Could you check a few things on this model? Use its own coordinates, in mm. A direction names the side the tool comes from. Round coordinates to 2 decimals unless told otherwise and drop trailing zeros. Loops run counter-clockwise (first coordinate to the right, second up) from the corner with the lowest first, then second, coordinate; pieces in that order, holes last. Notation, with made-up numbers: (59.5, 82.25) - (72.5, 82.25) arc R12 ccw to (72.5, 87.25) - close; hole circle Ø7 at (57, -32.5). An arc over 180 degrees is marked (long way). Use one line per item in the form item = value.
```python
from build123d import *

# Parameters (mm, degrees)
SKETCH1_W                = 51
SKETCH1_H                = 53.5
BOSS_EXTRUDE1_DEPTH      = 54.25
SKETCH2_W                = 43
SKETCH2_H                = 43
CUT_EXTRUDE1_DEPTH       = 50.75
SKETCH3_W                = 43
SKETCH3_H                = 3.5
CUT_EXTRUDE2_DEPTH       = 37.5
CUT_EXTRUDE3_DEPTH       = 76
SKETCH5_R                = 9.673114497
SKETCH5_R_2              = 5.390775308
SKETCH5_R_3              = 5.456912487
CUT_EXTRUDE4_DEPTH       = 76
SKETCH6_R                = 14
SKETCH6_R_2              = 1.75
CUT_EXTRUDE5_DEPTH       = 76
SKETCH7_R                = 5
CUT_EXTRUDE6_DEPTH       = 76
CUT_EXTRUDE7_DEPTH       = 27
FILLET2_R                = 1
SKETCH12_R               = 1.75
CUT_EXTRUDE8_DEPTH       = 15
BOSS_EXTRUDE4_DEPTH      = 10
BOSS_EXTRUDE4_DEPTH_BACK = 61
SKETCH13_W               = 16.75
SKETCH13_H               = 3.5
SKETCH14_W               = 71
SKETCH14_H               = 1.75
BOSS_EXTRUDE5_DEPTH      = 15
SKETCH15_R               = 1.75
CUT_EXTRUDE9_DEPTH       = 10
SKETCH16_R               = 1.75
CUT_EXTRUDE10_DEPTH      = 10
CUT_EXTRUDE11_REACH      = 95.245
FILLET3_R                = 5
FILLET4_R                = 1
CUT_EXTRUDE12_DEPTH      = 3


with BuildPart() as part:
    # Sketch1 → Boss-Extrude1 (new body)
    with BuildSketch(Plane.XY):
        with Locations((-26.432354029, 2.021717979)):
            Rectangle(SKETCH1_W, SKETCH1_H)
    extrude(amount=BOSS_EXTRUDE1_DEPTH)

    # Sketch2 → Cut-Extrude1 (cut)
    with BuildSketch(Plane.XY.offset(54.25)):
        with Locations((-26.432354029, 3.771717979)):
            Rectangle(SKETCH2_W, SKETCH2_H)
    extrude(amount=-CUT_EXTRUDE1_DEPTH, mode=Mode.SUBTRACT)

    # Sketch3 → Cut-Extrude2 (cut)
    with BuildSketch(Plane.XY.offset(54.25)):
        with Locations((-26.432354029, 27.021717979)):
            Rectangle(SKETCH3_W, SKETCH3_H)
    extrude(amount=-CUT_EXTRUDE2_DEPTH, mode=Mode.SUBTRACT)

    # Sketch4 → Cut-Extrude3 (cut)
    with BuildSketch(Plane.ZY.offset(51.932354029)):
        with BuildLine():
            Line((16.75, 28.771717979), (54.25, 28.771717979))
            Line((54.25, 28.771717979), (54.25, -7.074674815))
            ThreePointArc((54.25, -7.074674815), (27.422353926, 2.398250742), (16.75, 28.771717979))
        make_face()
    extrude(amount=-CUT_EXTRUDE3_DEPTH, mode=Mode.SUBTRACT)

    # Sketch5 → Cut-Extrude4 (cut)
    with BuildSketch(Plane.ZY.offset(51.932354029)):
        with Locations(Location((14.525222974, -6.808047023, 0), (0, 0, 270))):
            Circle(SKETCH5_R)
        with Locations(Location((34.168969833, -12.297713654, 0), (0, 0, 270))):
            Circle(SKETCH5_R_2)
        with Locations(Location((9.035556344, 13.166402645, 0), (0, 0, 270))):
            Circle(SKETCH5_R_3)
    extrude(amount=-CUT_EXTRUDE4_DEPTH, mode=Mode.SUBTRACT)

    # Sketch6 → Cut-Extrude5 (cut)
    with BuildSketch(Plane.XY.offset(3.5)):
        with Locations((-26.432354029, 3.771717979)):
            Circle(SKETCH6_R)
        with Locations((-10.932354029, 19.271717979)):
            Circle(SKETCH6_R_2)
        with Locations((-41.932354029, 19.271717979)):
            Circle(SKETCH6_R_2)
        with Locations((-41.932354029, -11.728282021)):
            Circle(SKETCH6_R_2)
        with Locations((-10.932354029, -11.728282021)):
            Circle(SKETCH6_R_2)
    extrude(amount=-CUT_EXTRUDE5_DEPTH, mode=Mode.SUBTRACT)

    # Sketch7 → Cut-Extrude6 (cut)
    with BuildSketch(Plane(origin=(0, 0, 0), x_dir=(-1, 0, 0), z_dir=(0, 0, -1))):
        with Locations((26.432354029, -24.728282021)):
            Circle(SKETCH7_R)
    extrude(amount=-CUT_EXTRUDE6_DEPTH, mode=Mode.SUBTRACT)

    # Sketch8 → Cut-Extrude7 (cut)
    with BuildSketch(Plane.XZ.offset(24.728282021)):
        Polygon((-26.432354029, 46.625), (-6.932354029, 27.125), (-26.432354029, 7.625), (-45.932354029, 27.125), align=None)
        Polygon((-13.361286217, 40.625), (-4.932354029, 40.625), (-4.932354029, 32.196067812), align=None)
        Polygon((-4.932354029, 13.625), (-13.361286217, 13.625), (-4.932354029, 22.053932188), align=None)
        Polygon((-47.932354029, 13.625), (-39.503421841, 13.625), (-47.932354029, 22.053932188), align=None)
        Polygon((-47.932354029, 40.625), (-39.007101497, 40.625), (-47.932354029, 31.699747468), align=None)
    extrude(amount=-CUT_EXTRUDE7_DEPTH, mode=Mode.SUBTRACT)

    # Fillet2
    fillet2_edges = [part.edges().sort_by_distance(p)[0] for p in [
        (-47.932354029, -21.228282021, 31.699747468),
        (-4.932354029, -21.228282021, 32.196067812),
        (-4.932354029, -21.228282021, 22.053932188),
        (-47.932354029, -21.228282021, 22.053932188),
        (-13.361286217, -21.228282021, 13.625),
        (-39.503421841, -21.228282021, 13.625),
        (-26.432354029, -18.728282021, 7.625),
        (-4.932354029, -21.228282021, 13.625),
        (-47.932354029, -21.228282021, 13.625),
        (-45.932354029, -21.228282021, 27.125),
        (-6.932354029, -21.228282021, 27.125),
        (-4.932354029, -21.228282021, 40.625),
        (-47.932354029, -21.228282021, 40.625),
        (-39.007101497, -21.228282021, 40.625),
        (-13.361286217, -21.228282021, 40.625),
        (-26.432354029, -18.728282021, 46.625),
    ]]
    fillet(fillet2_edges, radius=FILLET2_R)

    # Sketch12 → Cut-Extrude8 (cut)
    with BuildSketch(Plane.XZ.offset(24.728282021)):
        with Locations(Location((-11.432354029, 46.25, 0), (0, 0, 270))):
            Circle(SKETCH12_R)
        with Locations(Location((-41.432354029, 46.25, 0), (0, 0, 270))):
            Circle(SKETCH12_R)
        with Locations(Location((-11.432354029, 8, 0), (0, 0, 270))):
            Circle(SKETCH12_R)
        with Locations(Location((-41.432354029, 8, 0), (0, 0, 270))):
            Circle(SKETCH12_R)
    extrude(amount=-CUT_EXTRUDE8_DEPTH, mode=Mode.SUBTRACT)

    # Sketch13 → Boss-Extrude4 (add, two sides: drawn at the far end of the back side and taken through both)
    with BuildSketch(Plane.ZY.offset(51.932354029).offset(-BOSS_EXTRUDE4_DEPTH_BACK)):
        with Locations((8.375, 27.021717979)):
            Rectangle(SKETCH13_W, SKETCH13_H)
    extrude(amount=BOSS_EXTRUDE4_DEPTH + BOSS_EXTRUDE4_DEPTH_BACK)

    # Sketch14 → Boss-Extrude5 (add)
    with BuildSketch(Plane(origin=(0, 28.771717979, 0), x_dir=(1, 0, 0), z_dir=(0, 1, 0))):
        with Locations((-26.432354029, -0.875)):
            Rectangle(SKETCH14_W, SKETCH14_H)
    extrude(amount=BOSS_EXTRUDE5_DEPTH)

    # Sketch15 → Cut-Extrude9 (cut)
    with BuildSketch(Plane.XZ.offset(-25.271717979)):
        with Locations((-56.932354029, 9.25)):
            Circle(SKETCH15_R)
        with Locations((4.067645971, 9.25)):
            Circle(SKETCH15_R)
    extrude(amount=-CUT_EXTRUDE9_DEPTH, mode=Mode.SUBTRACT)

    # Sketch16 → Cut-Extrude10 (cut)
    with BuildSketch(Plane(origin=(0, 0, 0), x_dir=(-1, 0, 0), z_dir=(0, 0, -1))):
        with Locations((54.432354029, 36.271717979)):
            Circle(SKETCH16_R)
        with Locations((-1.567645971, 36.271717979)):
            Circle(SKETCH16_R)
        with Locations((44.432354029, 36.271717979)):
            Circle(SKETCH16_R)
        with Locations((8.432354029, 36.271717979)):
            Circle(SKETCH16_R)
    extrude(amount=-CUT_EXTRUDE10_DEPTH, mode=Mode.SUBTRACT)

    # Cut-Extrude11: up to this face of the body (flat: up to its plane)
    cut_extrude11_end = Plane(part.part.faces().sort_by_distance((-26.432354029, -17.120170189, 3.5))[0])
    # Sketch17 → Cut-Extrude11 (cut, up to the picked face)
    with BuildSketch(Plane.XY.offset(54.25), mode=Mode.PRIVATE) as cut_extrude11_sk1:
        with BuildLine():
            Line((-17.488082119, -19.228282021), (-4.932354029, -19.228282021))
            Line((-4.932354029, -19.228282021), (-4.932354029, -17.728282021))
            Line((-4.932354029, -17.728282021), (-18.606116108, -17.728282021))
            ThreePointArc((-18.606116108, -17.728282021), (-18.013624909, -18.453331822), (-17.488082119, -19.228282021))
        make_face()
    cut_extrude11_tool1 = split(extrude(cut_extrude11_sk1.sketch, amount=-CUT_EXTRUDE11_REACH, mode=Mode.PRIVATE), bisect_by=cut_extrude11_end, keep=Keep.BOTH, mode=Mode.PRIVATE)
    # Sketch17 → Cut-Extrude11 (cut, up to the picked face)
    with BuildSketch(Plane.XY.offset(54.25), mode=Mode.PRIVATE) as cut_extrude11_sk2:
        with BuildLine():
            Line((-35.376625939, -19.228282021), (-47.932354029, -19.228282021))
            Line((-47.932354029, -19.228282021), (-47.932354029, -17.728282021))
            Line((-47.932354029, -17.728282021), (-34.25859195, -17.728282021))
            ThreePointArc((-34.25859195, -17.728282021), (-34.851083149, -18.453331822), (-35.376625939, -19.228282021))
        make_face()
    cut_extrude11_tool2 = split(extrude(cut_extrude11_sk2.sketch, amount=-CUT_EXTRUDE11_REACH, mode=Mode.PRIVATE), bisect_by=cut_extrude11_end, keep=Keep.BOTH, mode=Mode.PRIVATE)
    add(cut_extrude11_tool1.solids().sort_by(Axis((-11.476334, -18.467624, 54.25), (0, 0, -1)))[0], mode=Mode.SUBTRACT)
    add(cut_extrude11_tool2.solids().sort_by(Axis((-41.388374, -18.467624, 54.25), (0, 0, -1)))[0], mode=Mode.SUBTRACT)

    # Fillet3
    fillet3_edges = [part.edges().sort_by_distance(p)[0] for p in [
        (-2.932354029, -7.074674815, 54.25),
        (-49.932354029, -7.074674815, 54.25),
    ]]
    fillet(fillet3_edges, radius=FILLET3_R)

    # Fillet4
    fillet4_edges = [part.edges().sort_by_distance(p)[0] for p in [
        (-51.932354029, 25.271717979, 8.375),
        (-0.932354029, 25.271717979, 8.375),
        (-0.932354029, -24.728282021, 27.125),
        (-51.932354029, -24.728282021, 27.125),
    ]]
    fillet(fillet4_edges, radius=FILLET4_R)

    # Sketch19 → Cut-Extrude12 (cut)
    with BuildSketch(Plane(origin=(0, -24.728282021, 0), x_dir=(1, 0, 0), z_dir=(0, 1, 0))):
        Polygon((-44.432354029, -9.732050808), (-41.432354029, -11.464101615), (-38.432354029, -9.732050808), (-38.432354029, -6.267949192), (-41.432354029, -4.535898385), (-44.432354029, -6.267949192), align=None)
        Polygon((-11.432354029, -4.535898385), (-14.432354029, -6.267949192), (-14.432354029, -9.732050808), (-11.432354029, -11.464101615), (-8.432354029, -9.732050808), (-8.432354029, -6.267949192), align=None)
        Polygon((-38.432354029, -47.982050808), (-38.432354029, -44.517949192), (-41.432354029, -42.785898385), (-44.432354029, -44.517949192), (-44.432354029, -47.982050808), (-41.432354029, -49.714101615), align=None)
        Polygon((-8.432354029, -47.982050808), (-8.432354029, -44.517949192), (-11.432354029, -42.785898385), (-14.432354029, -44.517949192), (-14.432354029, -47.982050808), (-11.432354029, -49.714101615), align=None)
    extrude(amount=CUT_EXTRUDE12_DEPTH, mode=Mode.SUBTRACT)


solid = part.part
```
1. If we section it at A-A, the plane y = 14: Write out the boundary of the cut face in (x, z).
Solution:
outline = (-51.93, 0) - (-35.99, 0) - (-35.99, 3.5) - (-47.93, 3.5) - (-47.93, 3.64) - (-51.93, 3.64) - close; (-51.93, 14.43) - (-47.93, 14.43) - (-47.93, 19.43) - (-51.93, 19.43) - close; (-16.87, 0) - (-0.93, 0) - (-0.93, 3.64) - (-4.93, 3.64) - (-4.93, 3.5) - (-16.87, 3.5) - close; (-4.93, 14.43) - (-0.93, 14.43) - (-0.93, 19.43) - (-4.93, 19.43) - close
2. If we section it at B-B, the plane y = 39: Write out the boundary of the cut face in (x, z).
Solution:
outline = (-61.93, 0) - (9.07, 0) - (9.07, 1.75) - (-61.93, 1.75) - close
3. We'd pull the mould along Z, two halves only. Please class faces 1 (the face through (-38.432, -23, 8)), 2 (the face through (-2.96, 2.86, 26.95)), 3 (the face through (-8.5, -19.228, 29.2)): +Z half, -Z half, draft (parallel to the pull), parting line (faces both ways), or undercut.
Solution:
face_1 = undercut
face_2 = +Z half
face_3 = draft
4. Please list where these lines run through material, in increasing order: line 1 along X through (y, z) = (5, 13); line 2 along Y through (x, z) = (-7.5, 12.5); line 3 along Z through (x, y) = (-6, 38).
Solution:
line_1 = -51.93 to -47.93, -4.93 to -0.93
line_2 = -24.73 to -19.23, 25.27 to 28.77
line_3 = 0 to 1.75
5. On a 3-axis mill with a long thin cutter (end or side, diameter ignored), from which of +Z, -Z, +X, -X, +Y, -Y can I reach the whole of each face in a straight line? I mean faces 4 (the face through (-43.68, -11.65, 1.77)), 5 (the face through (-43.43, -22.02, 36.2)), 6 (the face through (-51.932, -5, 27)), 7 (the face through (-2.96, -11.129, 28.906)), 8 (the face through (-10.1, -21.728, 9.5)). Say none if no direction works.
Solution:
face_4 = +Z, -Z
face_5 = +Y, -Y
face_6 = +Z, -Z, -X, -Y
face_7 = +X, -X
face_8 = -Y
6. For P1, Ø1.5, axis at y = -23.5, z = 45.5, coming from the -X side; P2, Ø4, axis at x = -21.5, z = 7.5, coming from the +Y side; P3, Ø15.5, axis at y = -6.81, z = 14.53, coming from the +X side; P4, Ø5.5, axis at x = -44.43, y = 36.27, coming from the +Z side, each with a flat end and sliding along its axis, tell me the tip position at first contact or that it passes through.
Solution:
P1 = -51.93
P2 = 28.77
P3 = through
P4 = 1.75
